Model file for the job. Use its own axes, mm. A direction names the side the tool comes from. Give positions to 0.01 mm unless a question says otherwise; leave off trailing zeros. Order: outer loops, then holes, each group sorted by start corner. A loop starts at its lowest first (then second) coordinate and runs counter-clockwise, first axis right, second up. Notation, with made-up numbers: (63.25, 55) -> (110.25, 55) arc R11 ccw to (110.25, 63) -> close; hole circle Ø8 at (45, -13.75). An arc over 180 degrees is marked (long way). Use CSV: the item, a comma, the result in double quotes. Start each with the question number.
1. Cut at C-C on x = -52. Give the number of separate pieces and of enclosed holes in the cut face, then the cut area to 3 significant figures.
2. Pull direction Z, two halves, no side cores. Call faces 1 (the flat face through (1, 0, -15)), 2 (the flat face through (-23, 4, 6.133)): released by +Z, released by -Z, zero draft, split by the parting line, or undercut.
3. 3-axis set-ups, long thin cutter, end or side, ignore diameter. For faces 3 (the flat face through (-23, 4, -2.933)), 4 (the flat face through (-28.3, 2, 33)), 5 (the flat face through (25, 10, 61)): which of +Z, -Z, +X, -X, +Y, -Y reach the whole face in a straight line?
4. Drop flat-ended pins along their axis: pin 1 (4 mm diameter, centred on x = 7, z = 8.5, fed in from +Y); pin 2 (5 mm diameter, centred on y = 5.5, z = 18, fed in from +X); pin 3 (3.5 mm diameter, centred on x = -5.5, y = 4.5, fed in from +Z); pin 4 (10 mm diameter, centred on x = 52, z = -9.5, fed in from -Y). Give the stop position or say it passes through.
5. Cut at B-B on z = 0. List the corners of the cut face in (x, y).
6. Wall check: line 1 (X direction, y = 4.7, z = 8.5); line 2 (Z direction, x = 7, y = 2.7); line 3 (X direction, y = 4.3, z = 8.5). Give the ranges that are in metal, low to high. Write a range as from..to.
7. Cut at A-A on x = 0. List the corners of the cut face in (y, z).
```python
from build123d import *

# Parameters (mm, degrees)
CUT_EXTRUDE1_DEPTH       = 4
SKETCH4_W                = 5.866666667
SKETCH4_H                = 3
SKETCH4_W_2              = 5.866666666
BOSS_EXTRUDE1_DEPTH      = 10
BOSS_EXTRUDE1_DEPTH_BACK = 63.5
SKETCH5_R                = 1.65
CUT_EXTRUDE2_DEPTH       = 11
SKETCH8_W                = 5.866666667
SKETCH8_H                = 3
SKETCH8_W_2              = 5.866666666
BOSS_EXTRUDE3_DEPTH      = 8


with BuildPart() as part:
    # Sketch1 → Revolve1 (revolve)
    with BuildSketch(Plane.XY):
        Polygon((0, 0), (63, 0), (69, 10), (65.501428863, 10), (61.301428863, 3), (0, 3), align=None)
    revolve(axis=Axis((0, 0, 0), (0, 1, 0)))

    # Sketch2 → Cut-Extrude1 (cut, through all)
    with BuildSketch(Plane(origin=(0, 3, 0), x_dir=(1, 0, 0), z_dir=(0, 1, 0))):
        with BuildLine():
            Line((-28.3, -12), (-28.3, -54.378076287))
            ThreePointArc((-28.3, -54.378076287), (0, -61.301428863), (28.3, -54.378076287))
            Line((28.3, -54.378076287), (28.3, -12))
            Line((28.3, -12), (-28.3, -12))
        make_face()
    extrude(amount=-CUT_EXTRUDE1_DEPTH, mode=Mode.SUBTRACT)

    # Sketch4 → Boss-Extrude1 (add, two sides)
    with BuildSketch(Plane(origin=(0, 0, 0), x_dir=(0, 0, -1), z_dir=(1, 0, 0))) as boss_extrude1_sk:
        with Locations((-9.066666666, 4.5)):
            Rectangle(SKETCH4_W, SKETCH4_H)
        with Locations((0, 4.5)):
            Rectangle(SKETCH4_W_2, SKETCH4_H)
        with Locations((9.066666666, 4.5)):
            Rectangle(SKETCH4_W, SKETCH4_H)
    extrude(amount=BOSS_EXTRUDE1_DEPTH)
    extrude(boss_extrude1_sk.sketch, amount=-BOSS_EXTRUDE1_DEPTH_BACK)

    # Sketch5 → Cut-Extrude2 (cut, through all)
    with BuildSketch(Plane(origin=(0, 0, 0), x_dir=(1, 0, 0), z_dir=(0, 1, 0))):
        with Locations((7, -8.5)):
            Circle(SKETCH5_R)
        with Locations((7, 8.5)):
            Circle(SKETCH5_R)
        with Locations((-52, 8.5)):
            Circle(SKETCH5_R)
        with Locations((-52, -8.5)):
            Circle(SKETCH5_R)
    extrude(amount=CUT_EXTRUDE2_DEPTH, mode=Mode.SUBTRACT)

    # Sketch8 → Boss-Extrude3 (add)
    with BuildSketch(Plane(origin=(10, 0, 0), x_dir=(0, 0, -1), z_dir=(1, 0, 0))):
        with Locations((-9.066666666, 4.5)):
            Rectangle(SKETCH8_W, SKETCH8_H)
        with Locations((0, 4.5)):
            Rectangle(SKETCH8_W_2, SKETCH8_H)
        with Locations((9.066666666, 4.5)):
            Rectangle(SKETCH8_W, SKETCH8_H)
    extrude(amount=BOSS_EXTRUDE3_DEPTH)


solid = part.part
```
Verdict:
1,separate pieces,"3"
1,enclosed holes,"0"
1,area,"318 mm^2"
2,face 1,"zero draft"
2,face 2,"undercut"
3,face 3,"+Y"
3,face 4,"+Y, -Y"
3,face 5,"+Z, -Z, +X, -X, +Y"
4,pin 1,"y = 6"
4,pin 2,"x = 65.5"
4,pin 3,"z = 66.53"
4,pin 4,"y = 0"
5,outline,"(-69, 10) -> (-63, 0) -> (63, 0) -> (69, 10) -> (65.5, 10) -> (61.3, 3) -> (18, 3) -> (18, 6) -> (-63.1, 6) -> (-65.5, 10) -> close"
6,line 1,"-65.27..-53.65, -50.35..5.35, 8.65..18, 61.74..65.27"
6,line 2,"-64.24..-10.15, -6.85..6.85, 10.15..12, 60.9..64.24"
6,line 3,"-65.03..-53.65, -50.35..5.35, 8.65..18, 61.5..65.03"
7,outline,"(0, -63) -> (10, -69) -> (10, -65.5) -> (3, -61.3) -> (3, -12) -> (6, -12) -> (6, -6.13) -> (3, -6.13) -> (3, -2.93) -> (6, -2.93) -> (6, 2.93) -> (3, 2.93) -> (3, 6.13) -> (6, 6.13) -> (6, 12) -> (0, 12) -> close; (0, 61.3) -> (3, 61.3) -> (10, 65.5) -> (10, 69) -> (0, 63) -> close"
